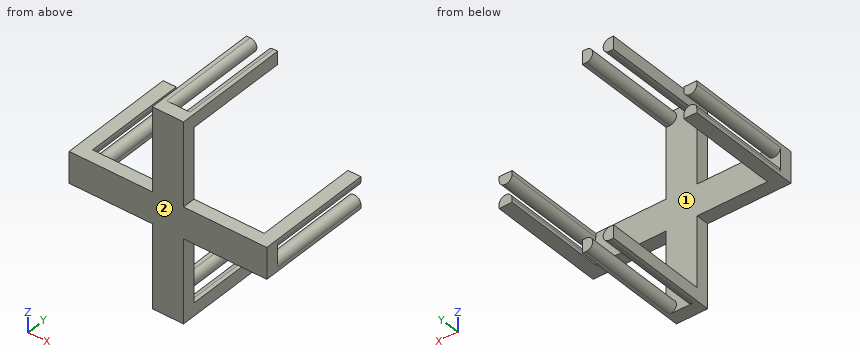
```python
from build123d import *

# Parameters (mm, degrees)
BOSS_EXTRUDE1_DEPTH = 2.5
BOSS_EXTRUDE2_DEPTH = 20
CIRPATTERN1_COUNT   = 4


with BuildPart() as part:
    # Sketch1 → Boss-Extrude1 (new body)
    with BuildSketch(Plane(origin=(0, 0, 0), x_dir=(1, 0, 0), z_dir=(0, 1, 0))):
        Polygon((-3, 3), (-3, 19), (3, 19), (3, 3), (19, 3), (19, -3), (3, -3), (3, -19), (-3, -19), (-3, -3), (-19, -3), (-19, 3), align=None)
    extrude(amount=BOSS_EXTRUDE1_DEPTH)

    # Sketch2 → Boss-Extrude2 (add)
    with BuildSketch(Plane(origin=(0, 2.5, 0), x_dir=(1, 0, 0), z_dir=(0, 1, 0))):
        with BuildLine():
            Line((-2.25, -19), (-3, -19))
            Line((-3, -19), (-3, -16.5))
            Line((-3, -16.5), (-2.25, -16.5))
            ThreePointArc((-2.25, -16.5), (-1, -17.75), (-2.25, -19))
        make_face()
        with BuildLine():
            Line((3, -16.5), (2.25, -16.5))
            ThreePointArc((2.25, -16.5), (1, -17.75), (2.25, -19))
            Line((2.25, -19), (3, -19))
            Line((3, -19), (3, -16.5))
        make_face()
    boss_extrude2 = extrude(amount=BOSS_EXTRUDE2_DEPTH)

    # CirPattern1: Boss-Extrude2 ×4 about axis
    cirpattern1_axis = Axis((0, 0, 0), (0, 1, 0))
    for i in range(1, CIRPATTERN1_COUNT):
        add(boss_extrude2.rotate(cirpattern1_axis, i * 360 / CIRPATTERN1_COUNT))


solid = part.part
```
CAD build for the part. Positions are in the model's coordinates, mm. Face numbers are marked on the shaded views. Round coordinates to 2 decimals unless told otherwise and drop trailing zeros. Write each loop counter-clockwise with the first axis right and the second up, starting at its lowest first coordinate (ties: lowest second). Pieces come first, ordered by that corner, then holes.
Item 1: Band-saw the part on D-D on z = 13.5. Write the cut outline in (x, y), then the cut area to 3 significant figures.
Filled in:
outline: (-3, 0) - (3, 0) - (3, 2.5) - (-3, 2.5) - close
area: 15.0 mm2
Item 2: Band-saw the part on C-C on x = 13. Write the cut outline in (y, z).
Filled in:
outline: (0, -3) - (2.5, -3) - (2.5, 3) - (0, 3) - close
Item 3: Mould opens along X. For the marked faces 1 and 2 say: released by +X, released by -X, zero draft, split by the parting line, or undercut.
Filled in:
face 1: undercut
face 2: zero draft
Item 4: Drop flat-ended pins along their axis: pin 1 Ø13 at (x, y) = (12.5, 12) entering from +Z; pin 2 Ø13 at (x, y) = (14.5, 15.5) entering from -Z; pin 3 Ø5 at (y, z) = (6.5, -13.5) entering from -X; pin 4 Ø5 at (y, z) = (5.5, 0.5) entering from -X. Give the stop position or say it passes through.
Filled in:
pin 1: stops at z = 3
pin 2: stops at z = -3
pin 3: passes through
pin 4: stops at x = -19
Item 5: Band-saw the part on A-A on y = 18.75. Give the number of separate pieces and of enclosed holes in the cut face, then the cut area to 3 significant figures.
Filled in:
separate pieces: 8
enclosed holes: 0
area: 34.6 mm2
Item 6: Band-saw the part on B-B on z = -17.75. Write the cut outline in (x, y), then the cut area to 3 significant figures.
Filled in:
outline: (-3, 0) - (3, 0) - (3, 22.5) - (1, 22.5) - (1, 2.5) - (-1, 2.5) - (-1, 22.5) - (-3, 22.5) - close
area: 95.0 mm2
Item 7: Drill centre lines: L1, parallel to Z at x = 17, y = 16.5; L2, parallel to X at y = 16, z = 1.5; L3, parallel to Z at x = 2, y = 18. Where is each one in solid material? Low to high.
Filled in:
L1: z = -3 to -1.25, 1.25 to 3
L2: x = -18.75 to -16.75, 16.75 to 18.75
L3: z = -18.97 to -16.53, 16.53 to 18.97
